Input: part model. Units: mm. Frame: model coordinates. A direction names the side the tool comes from. Round coordinates to 2 decimals unless told otherwise and drop trailing zeros. Loops run counter-clockwise (first coordinate to the right, second up) from the corner with the lowest first, then second, coordinate; pieces in that order, holes last. Notation, with made-up numbers: M 55.25,3 L 73.25,3 A24 ccw 73.25,36 Z; hole C 36.5,57 d7. An arc over 180 degrees is marked long. Use one line per item in the form item = value. Start each with the question number.
Q1. Section query A-A, the plane y = -2.55. Output: boundary loops of the cut face in (x, z), and give its area (3 significant figures).
Q2. Access query for faces 1 (the flat face through (-7.579, -2.5, -1.5)), 2 (the flat face through (-4.1, -3.5, 0)), 3 (the flat face through (7.579, -2.5, -1.5)), 4 (the flat face through (-4.1, -3.5, -3.997)). Directions: +Z, -Z, +X, -X, +Y, -Y. A direction counts if a zero-diameter tool reaches every point of the face in a straight line with its end or side. Return the directions, or none.
Q3. First-contact query: P1, Ø1.7, axis at y = -0.5, z = 16.5, coming from the +X side; P2, Ø1.1, axis at y = -3.5, z = -1.5, coming from the +X side; P3, Ø1.7, axis at y = -0.5, z = -13, coming from the +X side. Flat tips, straight axial feed; report the tip coordinate or a pass-through.
Q4. Section query C-C, the plane z = -11. Output: boundary loops of the cut face in (x, y), and give its area (3 significant figures).
Q5. Section query B-B, the plane x = -1.75. Output: boundary loops of the cut face in (y, z).
Q6. Mould query, pull axis X, two halves, no side actions, for faces 5 (the flat face through (10.5, -1, -12)), 6 (the flat face through (-2.472, -3.5, -2)), 7 (the flat face through (-1.216, -2.5, -1.5)), 8 (the flat face through (-4.4, -2.5, 5.379)). Classes: pulls with the +X half, pulls with the -X half, needs draft (parallel to the pull), parting line crosses it, or undercut.
Q7. Ray query, line 1 along Y through (x, z) = (7.5, 7); line 2 along Z through (x, y) = (6.5, -0.35); line 3 along X through (y, z) = (-0.95, -11.5). Return the intervals inside material, ascending.
Q8. Section query D-D, the plane x = -5. Output: boundary loops of the cut face in (y, z).
```python
from build123d import *

# Parameters (mm, degrees)
F2_DEPTH = 2.1
F1_W     = 6.362536
F1_H     = 13.562245
F1_W_2   = 3.264985
F1_H_2   = 3.997409
F3_DEPTH = 3
F4_DEPTH = 4


with BuildPart() as f2:
    # F0 (on Front) → F2 (new body)
    with BuildSketch(Plane.XZ):
        with BuildLine():
            Line((-10.5, 18.4), (-10.5, 9.26013))
            ThreePointArc((-10.5, 9.26013), (-14, 0), (-10.5, -9.26013))
            Line((-10.5, -9.26013), (-10.5, -18.4))
            Line((-10.5, -18.4), (0, -18.4))
            Line((0, -18.4), (0, -15.3))
            Line((0, -15.3), (10.5, -15.3))
            Line((10.5, -15.3), (10.5, -9.26013))
            ThreePointArc((10.5, -9.26013), (14, 0), (10.5, 9.26013))
            Line((10.5, 9.26013), (10.5, 15.3))
            Line((10.5, 15.3), (0, 15.3))
            Line((0, 15.3), (0, 18.4))
            Line((0, 18.4), (-10.5, 18.4))
        make_face()
    extrude(amount=F2_DEPTH)

    # F1 (on face) → F3 (join)
    with BuildSketch(Plane.XZ):
        with Locations((-4.397359, -1.402165)):
            Rectangle(F1_W, F1_H)
        with Locations((-4.104347, -1.998704)):
            Rectangle(F1_W_2, F1_H_2, mode=Mode.SUBTRACT)
        with Locations((4.397359, -1.402165)):
            Rectangle(F1_W, F1_H)
        with Locations((4.104347, -1.998704)):
            Rectangle(F1_W_2, F1_H_2, mode=Mode.SUBTRACT)
    extrude(amount=F3_DEPTH)

    # F1 (on face) → F4 (join)
    with BuildSketch(Plane.XZ):
        with Locations((-4.104347, -1.998704)):
            Rectangle(F1_W_2, F1_H_2)
        with Locations((4.104347, -1.998704)):
            Rectangle(F1_W_2, F1_H_2)
    extrude(amount=F4_DEPTH)


solid = f2.part
```
Results found:
q1.outline = M -7.58,-8.18 L -1.22,-8.18 L -1.22,5.38 L -7.58,5.38 Z; M 1.22,-8.18 L 7.58,-8.18 L 7.58,5.38 L 1.22,5.38 Z
q1.area = 173 mm²
q2.face_1 = +Z, -Z, -X, -Y
q2.face_2 = +Z, +X, -X, -Y
q2.face_3 = +Z, -Z, +X, -Y
q2.face_4 = -Z, +X, -X, -Y
q3.P1 = 0
q3.P2 = 7.58
q3.P3 = 10.5
q4.outline = M -10.5,-2.1 L 10.5,-2.1 L 10.5,0 L -10.5,0 Z
q4.area = 44.1 mm²
q5.outline = M -3,-8.18 L -2.1,-8.18 L -2.1,-18.4 L 0,-18.4 L 0,18.4 L -2.1,18.4 L -2.1,5.38 L -3,5.38 Z
q6.face_5 = pulls with the +X half
q6.face_6 = undercut
q6.face_7 = undercut
q6.face_8 = needs draft
q7.line_1 = -2.1 to 0
q7.line_2 = -15.3 to 15.3
q7.line_3 = -10.5 to 10.5
q8.outline = M -4,-4 L -3,-4 L -3,-8.18 L -2.1,-8.18 L -2.1,-18.4 L 0,-18.4 L 0,18.4 L -2.1,18.4 L -2.1,5.38 L -3,5.38 L -3,0 L -4,0 Z
